Read the model definition and answer for the solid it produces. Units are mm, in the model's axes. Coordinates: 2 decimals unless noted, no trailing zeros. Loops run counter-clockwise (first coordinate to the right, second up) from the corner with the lowest first, then second, coordinate; pieces in that order, holes last.
Q1. Section C-C (x = 380) is taken. Give the vertices of the cut face in (y, z).
Q2. Flat-ended cylindrical pins translate along their axes: P1, Ø10, axis at x = 453.5, y = 2.5, coming from the -Z side; P2, Ø1, axis at y = 5.5, z = 147, coming from the +X side; P3, Ø12, axis at x = 346, y = 4, coming from the -Z side; P4, Ø6, axis at x = 126, y = -3, coming from the +Z side. Find the tip coordinate at first contact, or state that the pin passes through.
Q3. Straight lines are drawn through the part: line 1 (X direction, y = -3.5, z = 226); line 2 (X direction, y = 3.5, z = 755); line 3 (Z direction, x = -64, y = 5). For each, find the intervals that lie inside material, in ascending order.
Q4. Section A-A (y = -3.5) is taken. Give the vertices of the cut face in (x, z).
Q5. Section B-B (z = 296) is taken. Give the vertices of the cut face in (x, y), then the cut area to 3 significant figures.
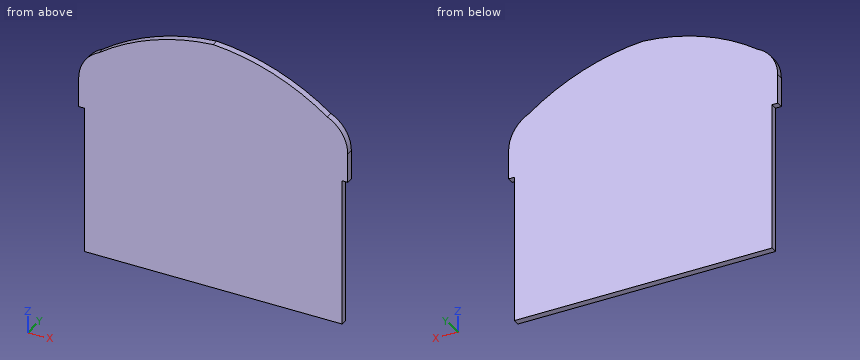
from build123d import *

# Parameters (mm, degrees)
SKETCH22_W          = 19.7612
SKETCH22_H          = 50.2412
BOSS_EXTRUDE3_DEPTH = 11.43


with BuildPart() as part:
    # Sketch22 → Boss-Extrude3 (new, symmetric)
    with BuildSketch(Plane(origin=(0, 0, 0), x_dir=(1, 0, 0), z_dir=(0, 1, 0))):
        with BuildLine():
            ThreePointArc((-393.602166776, -720.429950012), (-206.914351562, -819.647480117), (0, -863.039988079))
            ThreePointArc((0, -863.039988079), (206.914351562, -819.647480117), (393.602166776, -720.429950012))
            ThreePointArc((393.602166776, -720.429950012), (445.093816183, -675.319055068), (464.2612, -609.6))
            Line((464.2612, -609.6), (464.2612, -558.8))
            Line((464.2612, -558.8), (444.5, -558.8))
            Line((444.5, -558.8), (444.5, -508))
            Line((444.5, -508), (444.5, 0))
            Line((444.5, 0), (-444.5, 0))
            Line((-444.5, 0), (-444.5, -558.8))
            Line((-444.5, -558.8), (-464.2612, -558.8))
            Line((-464.2612, -558.8), (-464.2612, -609.6))
            ThreePointArc((-464.2612, -609.6), (-445.093816183, -675.319055068), (-393.602166776, -720.429950012))
        make_face()
        with Locations((454.3806, -533.6794)):
            Rectangle(SKETCH22_W, SKETCH22_H)
        with Locations((-454.3806, -533.6794)):
            Rectangle(SKETCH22_W, SKETCH22_H)
    extrude(amount=BOSS_EXTRUDE3_DEPTH, both=True)


solid = part.part
Numbers:
1. outline: (-11.43, 0) - (11.43, 0) - (11.43, 730.11) - (-11.43, 730.11) - close
2. P1: stops at z = 508.56
2. P2: stops at x = 444.5
2. P3: stops at z = 0
2. P4: stops at z = 844.64
3. line 1: x = -444.5 to 444.5
3. line 2: x = -341.74 to 341.74
3. line 3: z = 0 to 856.06
4. outline: (-464.26, 508.56) - (-444.5, 508.56) - (-444.5, 0) - (444.5, 0) - (444.5, 508.56) - (464.26, 508.56) - (464.26, 609.6) arc R122.25 ccw to (393.6, 720.43) arc R752.77 ccw to (0, 863.04) arc R752.77 ccw to (-393.6, 720.43) arc R122.25 ccw to (-464.26, 609.6) - close
5. outline: (-444.5, -11.43) - (444.5, -11.43) - (444.5, 11.43) - (-444.5, 11.43) - close
5. area: 20,300 mm2
